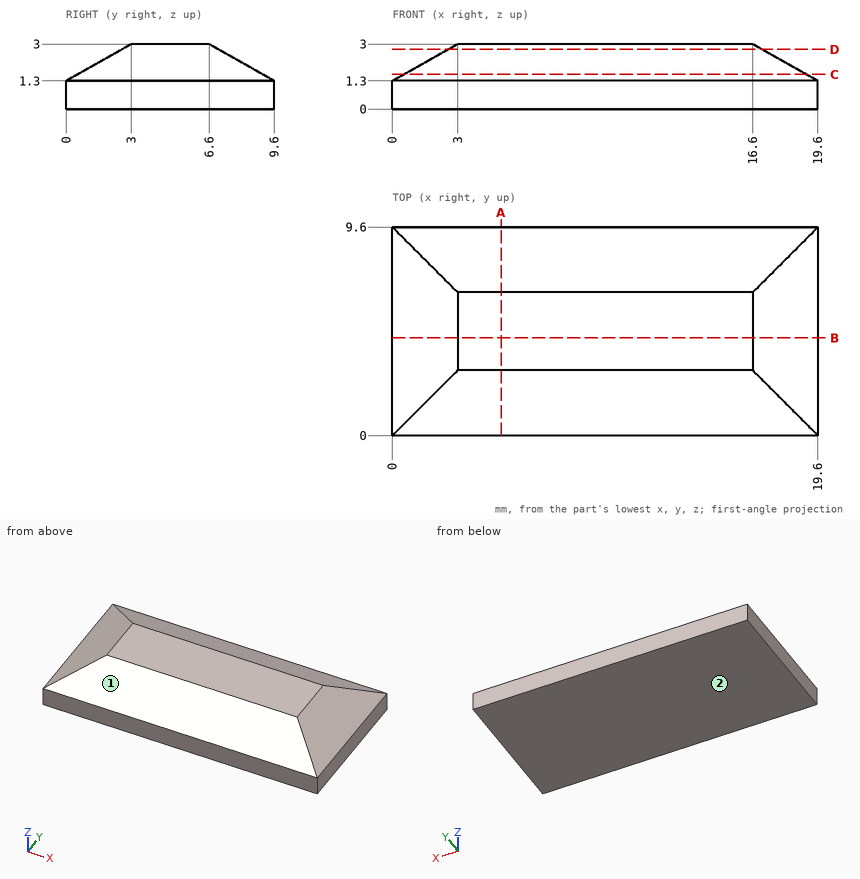
Input: dimensioned drawing with shaded views. Units: mm. Origin: part minimum x, y, z. Coordinates: 2 decimals unless noted, no trailing zeros. Order: outer loops, then holes, each group sorted by start corner. A loop starts at its lowest first (then second) coordinate and runs counter-clockwise, first axis right, second up.
1. Draft query along Y for the marked faces 1 and 2. Return one class per face: +Y half, -Y half, draft (parallel to the pull), parting line (faces both ways), or undercut.
Checked values:
face 1: -Y half
face 2: draft
2. Contact query for flat-ended pins moving along their axis: P1, Ø1, axis at x = 16, z = 2.5, coming from the +Y side; P2, Ø2, axis at x = 17, y = 2, coming from the +Z side; P3, Ø4, axis at x = 2, y = 2.5, coming from the -Z side. Output: stop coordinate, or through.
Checked values:
P1: stops at y = 8.36
P2: stops at z = 2.97
P3: stops at z = 0
3. Ray query, line 1 along Z through (x, y) = (17.5, 5.5); line 2 along Z through (x, y) = (18.75, 3.75); line 3 along X through (y, z) = (8, 2). Return the intervals inside material, ascending.
Checked values:
line 1: z = 0 to 2.49
line 2: z = 0 to 1.78
line 3: x = 1.24 to 18.36
4. Cut plane C-C, the plane z = 1.6. Return loops of the section in (x, y), plus the area to 3 significant figures.
Checked values:
outline: (0.53, 0.53) - (19.07, 0.53) - (19.07, 9.07) - (0.53, 9.07) - close
area: 158 mm2
5. Cut plane D-D, the plane z = 2.75. Return loops of the section in (x, y), plus the area to 3 significant figures.
Checked values:
outline: (2.56, 2.56) - (17.04, 2.56) - (17.04, 7.04) - (2.56, 7.04) - close
area: 64.9 mm2
6. Cut plane A-A, the plane x = 5. Return loops of the section in (y, z), plus the area to 3 significant figures.
Checked values:
outline: (0, 0) - (9.6, 0) - (9.6, 1.3) - (6.6, 3) - (3, 3) - (0, 1.3) - close
area: 23.7 mm2
7. Cut plane B-B, the plane y = 4.5. Return loops of the section in (x, z), plus the area to 3 significant figures.
Checked values:
outline: (0, 0) - (19.6, 0) - (19.6, 1.3) - (16.6, 3) - (3, 3) - (0, 1.3) - close
area: 53.7 mm2
